```python
from build123d import *

# Parameters (mm, degrees)
F0_W     = 342.9
F0_H     = 330.2
F1_DEPTH = 152.4
F2_W     = 317.5
F2_H     = 292.1
F3_DEPTH = 101.6
F4_R     = 9.525
F5_DEPTH = 69.85
F8_R     = 1.499997
F8_W     = 15.6979995019
F8_H     = 10.7923728456
F8_W_2   = 3.7969946861
F8_H_2   = 2.5979578495
F8_W_3   = 6.4112246037
F9_DEPTH = 25.4


with BuildPart() as f1:
    # F0 (on Top) → F1 (new body)
    with BuildSketch(Plane.XY):
        Rectangle(F0_W, F0_H)
    extrude(amount=F1_DEPTH)

    # F2 (on face) → F3 (cut)
    with BuildSketch(Plane.XY.offset(152.4)):
        with Locations((0, -6.35)):
            Rectangle(F2_W, F2_H)
    extrude(amount=-F3_DEPTH, mode=Mode.SUBTRACT)

    # F4 (on face) → F5 (cut, symmetric)
    with BuildSketch(Plane(origin=(0, 165.1, 0), x_dir=(-1, 0, 0), z_dir=(0, 1, 0))):
        with Locations((120.65, 50.8)):
            Circle(F4_R)
    extrude(amount=F5_DEPTH, both=True, mode=Mode.SUBTRACT)

    # F6 (on face) → F7 (revolve, cut)
    with BuildSketch(Plane.XY.offset(50.8)):
        with BuildLine():
            Line((-111.125, 95.25), (-130.175, 95.25))
            ThreePointArc((-130.175, 95.25), (-120.65, 85.725), (-111.125, 95.25))
        make_face()
    revolve(axis=Axis((-120.65, 95.25, 50.8), (1, 0, 0)), mode=Mode.SUBTRACT)

    # F8 (on face) → F9 (cut)
    with BuildSketch(Plane(origin=(0, -152.4, 0), x_dir=(-1, 0, 0), z_dir=(0, 1, 0))):
        with Locations((-107.869675722, 112.4142541665)):
            Circle(F8_R)
        with Locations((-107.9261657216, 120.1482748716)):
            Circle(F8_R)
        with Locations((-126.9230991602, 116.0683184862)):
            Rectangle(F8_W, F8_H)
        with Locations((-140.8484578133, 120.1762259007)):
            Rectangle(F8_W_2, F8_H_2)
        with Locations((-142.2262191772, 115.8662810922)):
            Rectangle(F8_W_3, F8_H_2)
        with Locations((-140.8484429121, 111.8389591575)):
            Rectangle(F8_W_2, F8_H_2)
    extrude(amount=-F9_DEPTH, mode=Mode.SUBTRACT)


solid = f1.part
```
Source: CAD feature listing. Evaluate the final solid. Frame: model axes, mm. A direction names the side the tool comes from. Coordinates: 2 decimals unless noted, no trailing zeros. Loops run counter-clockwise (first coordinate to the right, second up) from the corner with the lowest first, then second, coordinate; pieces in that order, holes last. Notation, with made-up numbers: (8.5, -13.75) -> (15.5, -13.75) arc R10 ccw to (15.5, -4.75) -> close; hole circle Ø11 at (43, 61.25). An arc over 180 degrees is marked (long way). One line per item, written item: value. Start each with the question number.
Q1. Line query: line 1 along Y through (x, z) = (148, 52.5); line 2 along X through (y, z) = (104, 119); line 3 along Z through (x, y) = (73, 77). Output: solid intervals per line, ascending.
Q2. Set-up query: faces 1 (the face through (-2, -165.1, 75)), 2 (the face through (-118.6, 138.4, 41.5)), 3 (the face through (-158.75, -8, 102)), 4 (the face through (127, -159, 110.672)), 5 (the face through (171.45, -2, 75)). Return all of +Z, -Z, +X, -X, +Y, -Y with unobstructed straight access to the full face (end or side cutting, diameter ignored); none if empty.
Q3. Section query C-C, the plane x = 18.5. Return the cut outline in (y, z).
Q4. Section query A-A, the plane x = -120.65. Return the cut outline in (y, z) (3 decimals), and give its area (3 significant figures).
Q5. Mould query, pull axis X, two halves, no side actions, for faces 6 (the face through (-1, 148, 152.4)), 7 (the face through (-171.45, -2, 75)), 8 (the face through (119.074, -159, 116)), 9 (the face through (-2, 139.7, 102)). Classes: pulls with the +X half, pulls with the -X half, needs draft (parallel to the pull), parting line crosses it, or undercut.
Q6. Section query B-B, the plane z = 132. Return the cut outline in (x, y).
Q7. Section query D-D, the plane y = -28.5. Return the cut outline in (x, z).
Results:
1. line 1: -165.1 to -152.4, 139.7 to 165.1
1. line 2: -171.45 to -158.75, 158.75 to 171.45
1. line 3: 0 to 50.8
2. face 1: +Z, -Z, +X, -X, -Y
2. face 2: +Y
2. face 3: +Z
2. face 4: -Y
2. face 5: +Z, -Z, +X, +Y, -Y
3. outline: (-165.1, 0) -> (165.1, 0) -> (165.1, 152.4) -> (139.7, 152.4) -> (139.7, 50.8) -> (-152.4, 50.8) -> (-152.4, 152.4) -> (-165.1, 152.4) -> close
4. outline: (-165.1, 0) -> (165.1, 0) -> (165.1, 41.275) -> (95.25, 41.275) arc R9.525 cw to (85.725, 50.8) -> (-152.4, 50.8) -> (-152.4, 152.4) -> (-165.1, 152.4) -> close; (139.7, 60.325) -> (165.1, 60.325) -> (165.1, 152.4) -> (139.7, 152.4) -> close
4. area: 19,700 mm^2
5. face 6: needs draft
5. face 7: pulls with the -X half
5. face 8: undercut
5. face 9: undercut
6. outline: (-171.45, -165.1) -> (171.45, -165.1) -> (171.45, 165.1) -> (-171.45, 165.1) -> close; hole (-158.75, -152.4) -> (158.75, -152.4) -> (158.75, 139.7) -> (-158.75, 139.7) -> close
7. outline: (-171.45, 0) -> (171.45, 0) -> (171.45, 152.4) -> (158.75, 152.4) -> (158.75, 50.8) -> (-158.75, 50.8) -> (-158.75, 152.4) -> (-171.45, 152.4) -> close
